Check sheet for the modelled part. Datum: model origin and axes. Units: mm. A direction names the side the tool comes from. Give positions to 0.01 mm unless a question says otherwise; leave off trailing zeros. Order: outer loops, then holes, each group sorted by start corner. A loop starts at its lowest first (then second) coordinate and runs counter-clockwise, first axis right, second up. Notation, with made-up numbers: M -33.5,-18 L 11.5,-18 A15 cw 11.5,-10 Z; hole C 35,-25 d8. An arc over 180 degrees is marked long. Return JSON: item names as keys, results as strings. Group by question number.
Solid Edge part; units mm, degrees
sketch "Sketch1" plane through (0, 0, 0) normal (0, 0, 1) x (1, 0, 0)
  line L0 (-60.5, -14) -> (60.5, -14)
  line L1 (60.5, -14) -> (60.5, 14)
  line L2 (60.5, 14) -> (-60.5, 14)
  line L3 (-60.5, 14) -> (-60.5, -14)
extrude "Protrusion1" add sketch "Sketch1" against normal blind 40
sketch "Sketch2" plane through (0, -14, -20) normal (0, -1, 0) x (1, 0, 0)
  line L0 (60.5, 20) -> (42, 20)
  line L1 (42, 20) -> (42, 11.5)
  line L2 (42, 11.5) -> (60.5, 11.5)
  line L3 (60.5, 11.5) -> (60.5, 20)
  line L4 (-60.5, 11.5) -> (-42, 11.5)
  line L5 (-42, 11.5) -> (-42, 20)
  line L6 (-42, 20) -> (-60.5, 20)
  line L7 (-60.5, 20) -> (-60.5, 11.5)
extrude "ExtrudedCutout_1" cut sketch "Sketch2" against normal blind 28
extrude "Cutout1" [suppressed]
sketch "Sketch3" plane through (0, 11.075, 0) normal (0, 0, 1) x (1, 0, 0)
  line L0 (60.5, -2.925) -> (60.5, 0)
  line L1 (60.5, 0) -> (42, -2.925)
  line L2 (42, -2.925) -> (60.5, -2.925)
  line L3 (60.5, -19.225) -> (60.5, -22.125)
  line L4 (60.5, -22.125) -> (42, -19.225)
  line L5 (42, -19.225) -> (60.5, -19.225)
  line L6 (-60.5, -2.925) -> (-60.5, 0)
  line L7 (-60.5, 0) -> (-42, -2.925)
  line L8 (-42, -2.925) -> (-60.5, -2.925)
  line L9 (-60.5, -19.225) -> (-60.5, -22.15)
  line L10 (-60.5, -22.15) -> (-42, -19.225)
  line L11 (-42, -19.225) -> (-60.5, -19.225)
extrude "ExtrudedCutout_4" cut sketch "Sketch3" against normal blind 33
sketch "Sketch4" plane through (0, 0, 0) normal (0, 0, 1) x (1, 0, 0)
  line L0 (-60.5, -8.3) -> (60.5, -8.3)
  line L1 (60.5, -8.3) -> (60.5, 8.3)
  line L2 (60.5, 8.3) -> (-60.5, 8.3)
  line L3 (-60.5, 8.3) -> (-60.5, -8.3)
extrude "ExtrudedCutout_5" cut sketch "Sketch4" against normal blind 33
chamfer "Chamfer_2" distance 3 distance2 18 1 edges at (-60.5, 0, -33) measured on face at (-60.5, 9.6133, -34.435)
chamfer "Chamfer_3" distance 3 distance2 18 1 edges at (60.5, 0.0125, -33) measured on face at (60.5, -9.6133, -34.435)
1) Material ranges on line 1 along Y through (x, z) = (28.5, -26); line 2 along Z through (x, y) = (-53.5, -12.5); line 3 along Z through (x, y) = (-34, -5.5), recorded low to high.
2) Sectioned sample at A-A on z = -28.5. Record the boundary of the cut face in (x, y) (3 decimals).
3) Sectioned sample at C-C on x = 27. Record the boundary of the cut face in (y, z).
4) Sectioned sample at D-D on y = -10. Record the boundary of the cut face in (x, z), then the cut area to 3 significant figures.
5) Tool access check on faces 1 (the face through (-51, 12, -8.5)), 2 (the face through (51, -12, -8.5)), 3 (the face through (-1, -8.3, -16)), 4 (the face through (51.9, -9.7, -22.1)), 5 (the face through (-51.8, -9.7, -22.1)). Record the directions out of +Z, -Z, +X, -X, +Y, -Y that give a thin tool (end or side, any length) a straight path to the whole face; none if there is none.
6) Sectioned sample at B-B on y = -3. Record the boundary of the cut face in (x, z).
7) Release check for a two-part mould opening along Y. For faces 6 (the face through (1, 14, -20)), 7 (the face through (-51.8, 9.7, -22.1)), 8 (the face through (60.5, 0, -37)), 9 (the face through (51.8, 9.7, -22.1)) record: released by +Y, released by -Y, zero draft, split by the parting line, or undercut.
8) Depth check by flat-ended pin: P1, Ø1.5, axis at x = -40.5, y = -6, coming from the +Z side; P2, Ø4.5, axis at x = -49, y = -10.5, coming from the +Z side; P3, Ø1.5, axis at y = -9.5, z = -7, coming from the -X side. Enter the tip coordinate at first touch or a pass-through.
Reply:
{
 "1": {"line 1": "-14 to -8.3, 8.3 to 14", "line 2": "-40 to -8.5", "line 3": "-40 to -33"},
 "2": {"outline": "M -60.5,-14 L 60.5,-14 L 60.5,-11.05 L 42.957,-8.3 L -42.949,-8.3 L -60.5,-11.075 Z; M -60.5,11.075 L -42.949,8.3 L 42.949,8.3 L 60.5,11.075 L 60.5,14 L -60.5,14 Z"},
 "3": {"outline": "M -14,-40 L 14,-40 L 14,0 L 8.3,0 L 8.3,-33 L -8.3,-33 L -8.3,0 L -14,0 Z"},
 "4": {"outline": "M -60.5,-40 L 60.5,-40 L 60.5,-36 L 53.8,-34.88 L 53.8,-8.5 L 42,-8.5 L 42,0 L -42,0 L -42,-8.5 L -53.7,-8.5 L -53.7,-34.87 L -60.5,-36 Z", "area": "4,160 mm^2"},
 "5": {"face 1": "+Z, -X, +Y, -Y", "face 2": "+Z, +X, +Y, -Y", "face 3": "+Z, +X, -X", "face 4": "+Z, +X", "face 5": "+Z, -X"},
 "6": {"outline": "M -60.5,-40 L 60.5,-40 L 60.5,-36 L 42.5,-33 L -42.5,-33 L -60.5,-36 Z"},
 "7": {"face 6": "released by +Y", "face 7": "undercut", "face 8": "zero draft", "face 9": "undercut"},
 "8": {"P1": "z = -33", "P2": "z = -8.5", "P3": "x = -42"}
}
